Work out the finished part from the listing and answer in its coordinate system (mm). Face numbers are marked on the shaded views. A direction names the side the tool comes from. Give positions to 0.01 mm unless a question says otherwise; leave off trailing zeros. Order: outer loops, then holes, each group sorted by start corner. A loop starts at its lowest first (then second) coordinate and runs counter-clockwise, first axis right, second up.
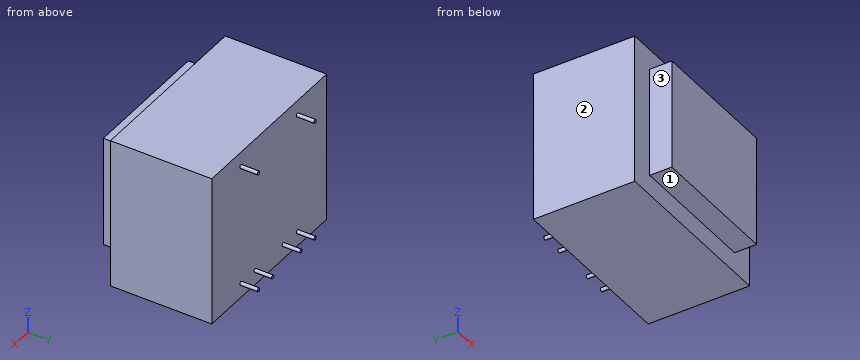
```python
from build123d import *

# Parameters (mm, degrees)
F0_W     = 40.6
F0_H     = 34.2
F1_DEPTH = 23
F2_W     = 30
F2_H     = 25
F3_DEPTH = 5
F4_R     = 0.4
F5_DEPTH = 4


with BuildPart() as f1:
    # F0 (on Front) → F1 (new body)
    with BuildSketch(Plane.XZ):
        Rectangle(F0_W, F0_H)
    extrude(amount=F1_DEPTH)

    # F2 (on face) → F3 (join)
    with BuildSketch(Plane.XZ.offset(23)):
        Rectangle(F2_W, F2_H)
    extrude(amount=F3_DEPTH)

    # F4 (on face) → F5 (join)
    with BuildSketch(Plane(origin=(0, 0, 0), x_dir=(-1, 0, 0), z_dir=(0, 1, 0))):
        with Locations((10, 13.75)):
            Circle(F4_R)
        with Locations((-10, 13.75)):
            Circle(F4_R)
        with Locations((-10, -13.75)):
            Circle(F4_R)
        with Locations((-5, -13.75)):
            Circle(F4_R)
        with Locations((10, -13.75)):
            Circle(F4_R)
        with Locations((5, -13.75)):
            Circle(F4_R)
    extrude(amount=F5_DEPTH)


solid = f1.part
```
1. Which of the six approach directions +Z, -Z, +X, -X, +Y, -Y give full straight-line access (tool end or side, diameter ignored) to the marked faces 1, 2 and 3?
Findings below:
face 1: -Z, +X, -X, -Y
face 2: +Z, -Z, -X, +Y, -Y
face 3: +Z, -Z, -X, -Y
2. Given P1, Ø3, axis at x = -4, z = 0.5, coming from the +Y side; P2, Ø2.5, axis at y = -25, z = 4, coming from the -X side; P3, Ø2.5, axis at x = -3.5, y = -26, coming from the +Z side, each flat-ended and moving along its own axis, determine where each tip first touches the part or whether it passes through.
Findings below:
P1: stops at y = 0
P2: stops at x = -15
P3: stops at z = 12.5
3. The part is cut by section D-D (z = -15). Write down the section's boundary in (x, y), then the cut area to 3 significant figures.
Findings below:
outline: (-20.3, -23) - (20.3, -23) - (20.3, 0) - (-20.3, 0) - close
area: 934 mm2
4. The part is cut by section A-A (z = -4). Write down the section's boundary in (x, y).
Findings below:
outline: (-20.3, -23) - (-15, -23) - (-15, -28) - (15, -28) - (15, -23) - (20.3, -23) - (20.3, 0) - (-20.3, 0) - close
5. Straight lines are drawn through the part: probe 1 along Y at (x, z) = (-13, -15); probe 2 along Y at (x, z) = (10, -8); probe 3 along X at (y, z) = (-26, 11.5). For each, find the intervals that lie inside material, in ascending order.
Findings below:
probe 1: y = -23 to 0
probe 2: y = -28 to 0
probe 3: x = -15 to 15
6. The part is cut by section B-B (x = 13). Write down the section's boundary in (y, z), then the cut area to 3 significant figures.
Findings below:
outline: (-28, -12.5) - (-23, -12.5) - (-23, -17.1) - (0, -17.1) - (0, 17.1) - (-23, 17.1) - (-23, 12.5) - (-28, 12.5) - close
area: 912 mm2
7. The part is cut by section C-C (y = -26). Write down the section's boundary in (x, z), then the cut area to 3 significant figures.
Findings below:
outline: (-15, -12.5) - (15, -12.5) - (15, 12.5) - (-15, 12.5) - close
area: 750 mm2
